Input: dimensioned drawing with shaded views. Units: mm. Origin: part minimum x, y, z. Give positions to 0.01 mm unless a question says otherwise; leave off trailing zeros. Loops run counter-clockwise (first coordinate to the right, second up) from the corner with the lowest first, then second, coordinate; pieces in that order, holes last. Notation, with made-up numbers: M -9,-12 L -3,-12 A25 ccw -3,4 Z; hole C -1,38.5 d11. An arc over 180 degrees is marked long. Use CSV: the item, a comma, the result in double quotes. Start each with the question number.
Q1. Section D-D, the plane y = 3.4. Output: boundary loops of the cut face in (x, z), plus the area to 3 significant figures.
Q2. Section B-B, the plane x = 5. Output: boundary loops of the cut face in (y, z), plus the area to 3 significant figures.
Q3. Material intervals for line 1 along X through (y, z) = (1.35, 17.5); line 2 along Z through (x, y) = (5, 1.55); line 3 along Y through (x, z) = (13, 63), sorted ascending.
Q4. Pin query (flat end, axial travel): pin 1 (4.5 mm diameter, centred on x = 95, z = 52.5, fed in from +Y); pin 2 (2 mm diameter, centred on y = 3.5, z = 43.5, fed in from +X); pin 3 (6.5 mm diameter, centred on x = 5, z = 17.5, fed in from +Y); pin 4 (1 mm diameter, centred on x = 40, y = 3, fed in from +Z). Return the tip coordinate at first contact, or that it passes through.
Q5. Section A-A, the plane z = 52.5. Output: boundary loops of the cut face in (x, y), plus the area to 3 significant figures.
Q6. Section C-C, the plane x = 51. Output: boundary loops of the cut face in (y, z).
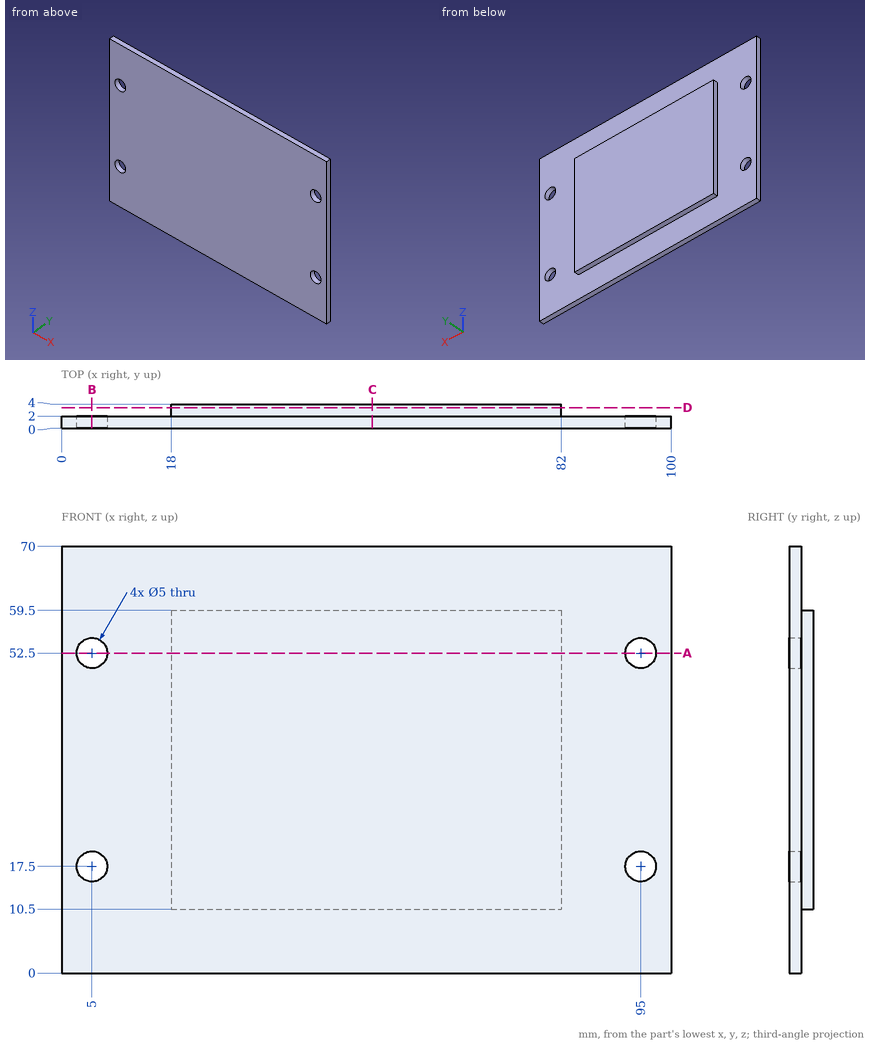
A:
1,outline,"M 18,10.5 L 82,10.5 L 82,59.5 L 18,59.5 Z"
1,area,"3,140 mm^2"
2,outline,"M 0,0 L 2,0 L 2,15 L 0,15 Z; M 0,20 L 2,20 L 2,50 L 0,50 Z; M 0,55 L 2,55 L 2,70 L 0,70 Z"
2,area,"120 mm^2"
3,line 1,"0 to 2.5, 7.5 to 92.5, 97.5 to 100"
3,line 2,"0 to 15, 20 to 50, 55 to 70"
3,line 3,"0 to 2"
4,pin 1,"through"
4,pin 2,"x = 82"
4,pin 3,"y = 2"
4,pin 4,"z = 59.5"
5,outline,"M 0,0 L 2.5,0 L 2.5,2 L 0,2 Z; M 7.5,0 L 92.5,0 L 92.5,2 L 82,2 L 82,4 L 18,4 L 18,2 L 7.5,2 Z; M 97.5,0 L 100,0 L 100,2 L 97.5,2 Z"
5,area,"308 mm^2"
6,outline,"M 0,0 L 2,0 L 2,10.5 L 4,10.5 L 4,59.5 L 2,59.5 L 2,70 L 0,70 Z"
